```python
from build123d import *

# Parameters (mm, degrees)
F0_R     = 206.5196172612
F0_R_2   = 1.7272
F1_DEPTH = 6.35
F2_R     = 6.34999


# Not quite as in the source:
# - a fillet or chamfer is up to 0.001 mm smaller than in the source, because OpenCascade refuses the exact size


with BuildPart() as f1:
    # F0 (on Top) → F1 (new body)
    with BuildSketch(Plane.XY):
        Circle(F0_R)
        with Locations((-96.9098086306, -167.8527123)):
            Circle(F0_R_2, mode=Mode.SUBTRACT)
        with Locations((96.9098086306, -167.8527123)):
            Circle(F0_R_2, mode=Mode.SUBTRACT)
        with Locations((-193.8196172612, 0)):
            Circle(F0_R_2, mode=Mode.SUBTRACT)
        with Locations((-96.9098086306, 167.8527123)):
            Circle(F0_R_2, mode=Mode.SUBTRACT)
        with Locations((193.8196172612, 0)):
            Circle(F0_R_2, mode=Mode.SUBTRACT)
        with Locations((96.9098086306, 167.8527123)):
            Circle(F0_R_2, mode=Mode.SUBTRACT)
    extrude(amount=F1_DEPTH)

    # F2 (radius 6.35 in the source; OpenCascade refuses exactly that, so slightly less here)
    f2_edges = [f1.edges().sort_by_distance(p)[0] for p in [
        (-206.519617, 0, 6.35),
    ]]
    fillet(f2_edges, radius=F2_R)


solid = f1.part
```
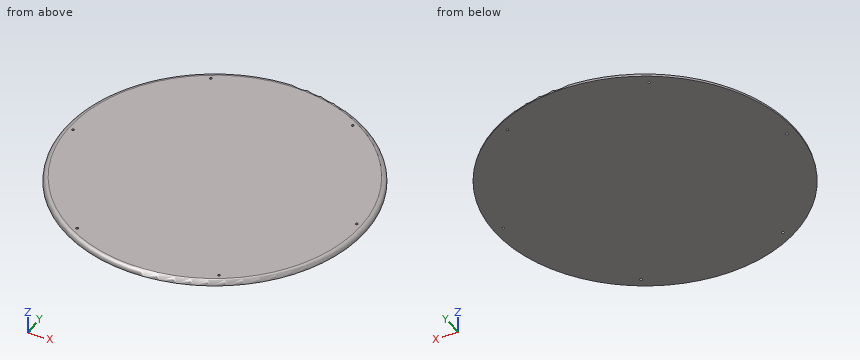
Can you work these out from the model? Positions are in its coordinate system, mm. Coordinates: 2 decimals unless noted, no trailing zeros. Loops run counter-clockwise (first coordinate to the right, second up) from the corner with the lowest first, then second, coordinate; pieces in that order, holes last.
1) Imagine slicing it at A-A on z = 3.75. List the corners of the cut face in (x, y) for me, plus the area to 3 significant figures.
2) For pin 1 (2 mm diameter, centred on x = -74, z = 3, fed in from -Y); pin 2 (1 mm diameter, centred on y = -119, z = 5.5, fed in from +X); pin 3 (2 mm diameter, centred on x = 154.5, z = 5.5, fed in from -Y), each with a flat end and sliding along its axis, tell me the tip position at first contact or that it passes through.
3) I need wall thicknesses on probe 1 along Y at (x, z) = (-158, 4.5); probe 2 along X at (y, z) = (55, 1.75); probe 3 along X at (y, z) = (35.5, 1). Which ranges of each line are inside material? Lowest first, please.
Completed:
1. outline: circle Ø410.59 at (0, 0); hole circle Ø3.45 at (-193.82, 0); hole circle Ø3.45 at (-96.91, -167.85); hole circle Ø3.45 at (-96.91, 167.85); hole circle Ø3.45 at (96.91, -167.85); hole circle Ø3.45 at (96.91, 167.85); hole circle Ø3.45 at (193.82, 0)
1. area: 132,000 mm2
2. pin 1: stops at y = -192.62
2. pin 2: stops at x = 165.88
2. pin 3: stops at y = -134.58
3. probe 1: y = -130.07 to 130.07
3. probe 2: x = -198.81 to 198.81
3. probe 3: x = -203.37 to 203.37
